Read the model definition and answer for the solid it produces. Units are mm, in the model's axes. Coordinates: 2 decimals unless noted, no trailing zeros. Answer as a JSON object with one key per item and string values. Group by question number.
from build123d import *

# Parameters (mm, degrees)
SKETCH1_R           = 2.1
BOSS_EXTRUDE1_DEPTH = 448


with BuildPart() as part:
    # Sketch1 → Boss-Extrude1 (new body)
    with BuildSketch(Plane.XY):
        Polygon((0, 0), (0, 5.36), (1.8, 7.16), (1.8, 4.500660172), (3.44, 4.500660172), (6.099339828, 7.16), (6.099339828, 12.84), (3.44, 15.499339828), (1.8, 15.499339828), (1.8, 12.84), (0, 14.64), (0, 20), (5.36, 20), (7.16, 18.2), (4.500660172, 18.2), (4.500660172, 16.56), (7.16, 13.900660172), (12.84, 13.900660172), (15.499339828, 16.56), (15.499339828, 18.2), (12.84, 18.2), (14.64, 20), (20, 20), (25.36, 20), (27.16, 18.2), (24.500939946, 18.2), (24.50125838, 16.559689577), (27.161114417, 13.900866058), (32.84111431, 13.901968719), (35.499937829, 16.561824756), (35.49961981, 18.2), (32.84, 18.2), (34.64, 20), (39.999930631, 20), (40.000970647, 14.642698508), (38.201320116, 12.842349107), (38.200803857, 15.501688885), (36.560803888, 15.501370511), (33.901980368, 12.841514474), (33.903083029, 7.161514581), (36.562939066, 4.502691062), (38.202939036, 4.503009436), (38.202422777, 7.162349214), (40.002772178, 5.362698683), (40.003813241, 0), (34.64, 0), (32.84, 1.8), (35.502803549, 1.8), (35.502484821, 3.441825004), (32.842628784, 6.100648523), (27.162628891, 6.099545862), (24.503805372, 3.439689825), (24.504123686, 1.8), (27.16, 1.8), (25.36, 0), (20, 0), (14.64, 0), (12.84, 1.8), (15.499339828, 1.8), (15.499339828, 3.44), (12.84, 6.099339828), (7.16, 6.099339828), (4.500660172, 3.44), (4.500660172, 1.8), (7.16, 1.8), (5.36, 0), align=None)
        with Locations((10, 10)):
            Circle(SKETCH1_R, mode=Mode.SUBTRACT)
        with Locations((30, 10)):
            Circle(SKETCH1_R, mode=Mode.SUBTRACT)
        Polygon((17.300660172, 3.76), (17.300660172, 1.8), (22.700660172, 1.8), (22.700660172, 3.76), (26.100660172, 7.16), (26.100660172, 12.84), (22.699339828, 16.24), (22.699339828, 18.2), (17.300660172, 18.2), (17.300660172, 16.24), (13.900660172, 12.84), (13.900660172, 7.16), align=None, mode=Mode.SUBTRACT)
        Polygon((1.8, 18.2), (3.430660172, 18.2), (3.430660172, 17.63), (2.37, 16.569339828), (1.8, 16.569339828), align=None, mode=Mode.SUBTRACT)
        Polygon((1.8, 3.430660172), (1.8, 1.8), (3.430660172, 1.8), (3.430660172, 2.37), (2.37, 3.430660172), align=None, mode=Mode.SUBTRACT)
        Polygon((38.2, 1.8), (36.569339828, 1.8), (36.569339828, 2.37), (37.63, 3.430660172), (38.2, 3.430660172), align=None, mode=Mode.SUBTRACT)
        Polygon((38.2, 16.569339828), (38.2, 18.2), (36.569339828, 18.2), (36.569339828, 17.63), (37.63, 16.569339828), align=None, mode=Mode.SUBTRACT)
    extrude(amount=-BOSS_EXTRUDE1_DEPTH)


solid = part.part
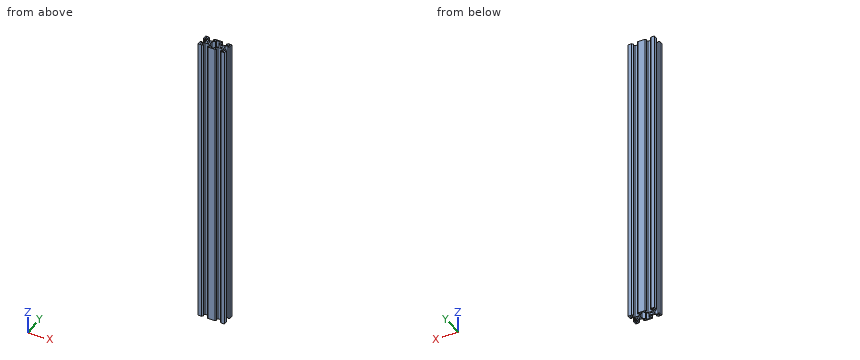
1. A cutting plane is placed at A-A on z = -403. State how many separate pieces and enclosed holes the cut face has, and give its area (3 significant figures).
2. Straight lines are drawn through the part: L1, parallel to Y at x = 10, z = -162; L2, parallel to X at y = 17.25, z = -156; L3, parallel to Y at x = 21.5, z = -315.5. For each, find the intervals that lie inside material, in ascending order.
3. Given pin 1 (0.8 mm diameter, centred on x = 34.5, z = -123, fed in from -Y); pin 2 (1.7 mm diameter, centred on y = 11, z = -275.5, fed in from +X); pin 3 (1.8 mm diameter, centred on y = 17.5, z = -125, fed in from +X); pin 4 (1.5 mm diameter, centred on x = 12, z = -188.5, fed in from +Y), each flat-ended and moving along its own axis, determine where each tip first touches the part or whether it passes through.
Derived:
{
 "1": {"separate pieces": "1", "enclosed holes": "7", "area": "292 mm2"},
 "2": {"L1": "y = 6.1 to 7.9, 12.1 to 13.9", "L2": "x = 0 to 1.8, 3.05 to 4.5, 15.5 to 17.3, 22.7 to 24.5, 35.5 to 36.95, 38.2 to 40", "L3": "y = 0 to 1.8, 18.2 to 20"},
 "3": {"pin 1": "stops at y = 0", "pin 2": "stops at x = 33.9", "pin 3": "stops at x = 40", "pin 4": "stops at y = 13.9"}
}
